The model under review builds one solid part; all positions refer to its coordinate system, in mm. Give positions to 0.01 mm unless a question says otherwise; leave off trailing zeros. Write each loop counter-clockwise with the first axis right and the second up, starting at its lowest first coordinate (ties: lowest second). Pieces come first, ordered by that corner, then holes. Notation, with made-up numbers: (59, -39.75) -> (76, -39.75) arc R29 ccw to (76, -14.75) -> close; hole circle Ø1 at (-17, 40.5). An arc over 180 degrees is marked (long way). Use CSV: the item, a comma, the result in double quotes.
```python
from build123d import *

# Parameters (mm, degrees)
SKETCH_1_W      = 1.2
SKETCH_1_H      = 7.2
SKETCH_1_H_2    = 7
SKETCH_1_R      = 0.5
EXTRUDE_1_DEPTH = 2
FILLET_1_R      = 0.5


with BuildPart() as part:
    # 草图1 → 凸台-拉伸1 (new body)
    # profile 1 of 2: a face of its own
    with BuildSketch(Plane(origin=(0, 0, 0), x_dir=(1, 0, 0), z_dir=(0, 1, 0))):
        with Locations((0, 8.6)):
            Rectangle(SKETCH_1_W, SKETCH_1_H)
    # profile 2 of 2: a face of its own
    with BuildSketch(Plane(origin=(0, 0, 0), x_dir=(1, 0, 0), z_dir=(0, 1, 0))):
        with Locations((0, 1.5)):
            Rectangle(SKETCH_1_W, SKETCH_1_H_2)
        with Locations(Location((0, 0, 0), (0, 0, 270))):
            Circle(SKETCH_1_R, mode=Mode.SUBTRACT)
    extrude(amount=EXTRUDE_1_DEPTH)

    # 圆角1
    fillet_1_edges = [part.edges().sort_by_distance(p)[0] for p in [
        (0, 2, -12.2),
        (0, 0, -12.2),
    ]]
    fillet(fillet_1_edges, radius=FILLET_1_R)


solid = part.part
```
Q1. The part is to be moulded in two halves that separate along Z. For faces 1 (the flat face through (0, 1, -12.2)), 2 (the flat face through (0.6, 1, -5)), 3 (the cylindrical face through (-0.3, 1, -0.4)), say which applies: pulls with the +Z half, pulls with the -Z half, needs draft (parallel to the pull), parting line crosses it, or undercut.
Derived:
face 1,"pulls with the -Z half"
face 2,"needs draft"
face 3,"undercut"
Q2. Consider section A-A (x = 0.3). Write out the cut boundary in (y, z), then the cut area to 3 significant figures.
Derived:
outline,"(0, -11.7) arc R0.5 ccw to (0.5, -12.2) -> (1.5, -12.2) arc R0.5 ccw to (2, -11.7) -> (2, -0.4) -> (0, -0.4) -> close; (0, 0.4) -> (2, 0.4) -> (2, 2) -> (0, 2) -> close"
area,"26.7 mm2"
Q3. Consider section B-B (z = 0). Write out the cut boundary in (x, y).
Derived:
outline,"(-0.6, 0) -> (-0.5, 0) -> (-0.5, 2) -> (-0.6, 2) -> close; (0.5, 0) -> (0.6, 0) -> (0.6, 2) -> (0.5, 2) -> close"
Q4. To check wall thickness, follow probe 1 along Z at (x, y) = (-0.05, 1.05); probe 2 along Z at (x, y) = (-0.25, 0.6). State the ranges of each line that lie inside material, in increasing order.
Derived:
probe 1,"z = -12.2 to -0.5, 0.5 to 2"
probe 2,"z = -12.2 to -0.43, 0.43 to 2"
Q5. Consider section C-C (x = -0.25). Write out the cut boundary in (y, z).
Derived:
outline,"(0, -11.7) arc R0.5 ccw to (0.5, -12.2) -> (1.5, -12.2) arc R0.5 ccw to (2, -11.7) -> (2, -0.43) -> (0, -0.43) -> close; (0, 0.43) -> (2, 0.43) -> (2, 2) -> (0, 2) -> close"
